```python
from build123d import *

# Parameters (mm, degrees)
F1_DEPTH = 50
F2_R     = 24.99999
F3_R     = 15.1938434026
F4_DEPTH = 73.4817621135
F5_R     = 5
F6_DEPTH = 38.6612540378


# Not quite as in the source:
# - a fillet or chamfer is up to 0.001 mm smaller than in the source, because OpenCascade refuses the exact size


with BuildPart() as f1:
    # F0 (on Top) → F1 (new body)
    with BuildSketch(Plane.XY):
        Polygon((0, 29.6784242139), (-80, 29.6784242139), (-80, 19.6784242139), (-2.6794919243, 19.6784242139), (46.9615242271, -8.9818298239), (51.9615242271, -0.3215757861), align=None)
    extrude(amount=F1_DEPTH)

    # F2 (radius 25 in the source; OpenCascade refuses exactly that, so slightly less here)
    f2_edges = [f1.edges().sort_by_distance(p)[0] for p in [
        (49.461524, -4.651703, 50),
        (49.461524, -4.651703, 0),
    ]]
    fillet(f2_edges, radius=F2_R)

    # F3 (on face) → F4 (cut, through all)
    with BuildSketch(Plane(origin=(12.8511346568, 22.2588181604, 0), x_dir=(-0.8660254038, 0.5, 0), z_dir=(0.5, 0.8660254038, 0))):
        with Locations((-20.160787893, 25)):
            Circle(F3_R)
    extrude(amount=-F4_DEPTH, mode=Mode.SUBTRACT)

    # F5 (on face) → F6 (cut, through all)
    with BuildSketch(Plane(origin=(0, 29.6784242139, 0), x_dir=(-1, 0, 0), z_dir=(0, 1, 0))):
        with Locations((12, 40)):
            Circle(F5_R)
        with Locations((70, 40)):
            Circle(F5_R)
        with Locations((12, 10)):
            Circle(F5_R)
        with Locations((70, 10)):
            Circle(F5_R)
    extrude(amount=-F6_DEPTH, mode=Mode.SUBTRACT)


solid = f1.part
```
Geometry: final body of the model. Coordinates: model frame, mm. A direction names the side the tool comes from. Coordinates: 2 decimals unless noted, no trailing zeros. Order: outer loops, then holes, each group sorted by start corner. A loop starts at its lowest first (then second) coordinate and runs counter-clockwise, first axis right, second up. Notation, with made-up numbers: (13.5, -8) -> (53.5, -8) arc R7 cw to (53.5, 5) -> close; hole circle Ø6 at (85, 20). An arc over 180 degrees is marked (long way). Write item = value, one per line.
(1) Pull-direction query (Z, two-part tool) for faces 1 (the flat face through (14.797, 21.135, 24.65)), 2 (the cylindrical face through (43.32, -1.03, 42.48)), 3 (the cylindrical face through (-74.619, 24.748, 8.085)); classes: pulls with the +Z half, pulls with the -Z half, needs draft (parallel to the pull), parting line crosses it, or undercut.
Solved:
face_1 = needs draft
face_2 = pulls with the +Z half
face_3 = undercut
(2) Line query: line 1 (Z direction, x = -70, y = 23); line 2 (Y direction, x = -28.5, z = 17.5); line 3 (Y direction, x = 13, z = 48.5). Output: solid intervals per line, ascending.
Solved:
line_1 = 0 to 5, 15 to 35, 45 to 50
line_2 = 19.68 to 29.68
line_3 = 10.63 to 22.17
(3) Cut plane A-A on x = -12. Return loops of the section in (y, z), plus the area to 3 significant figures.
Solved:
outline = (19.68, 0) -> (29.68, 0) -> (29.68, 5) -> (19.68, 5) -> close; (19.68, 15) -> (29.68, 15) -> (29.68, 35) -> (19.68, 35) -> close; (19.68, 45) -> (29.68, 45) -> (29.68, 50) -> (19.68, 50) -> close
area = 300 mm²
(4) Cut plane D-D on x = -63.5. Return loops of the section in (y, z), plus the area to 3 significant figures.
Solved:
outline = (19.68, 0) -> (29.68, 0) -> (29.68, 50) -> (19.68, 50) -> close
area = 500 mm²
(5) Access query for faces 4 (the flat face through (-26, 23, 0)), 5 (the flat face through (-42, 19.678, 25)). Directions: +Z, -Z, +X, -X, +Y, -Y. A direction counts if a zero-diameter tool reaches every point of the face in a straight line with its end or side. Return the directions, or none.
Solved:
face_4 = -Z, +X, -X, +Y, -Y
face_5 = +Z, -Z, -X, -Y
(6) Cut plane B-B on z = 18.5. Return loops of the section in (x, y).
Solved:
outline = (-80, 19.68) -> (-2.68, 19.68) -> (13.42, 10.38) -> (18.42, 19.05) -> (0, 29.68) -> (-80, 29.68) -> close; (37.2, -3.35) -> (46.22, -8.55) -> (51.22, 0.11) -> (42.2, 5.31) -> close
(7) Cut plane C-C on y = 24.5. Return loops of the section in (x, z).
Solved:
outline = (-80, 0) -> (8.97, 0) -> (8.97, 50) -> (-80, 50) -> close; hole circle Ø10 at (-70, 10); hole circle Ø10 at (-70, 40); hole circle Ø10 at (-12, 10); hole circle Ø10 at (-12, 40)
(8) Pin query (flat end, axial travel): pin 1 Ø13 at (x, z) = (-70, 10) entering from -Y; pin 2 Ø1 at (y, z) = (-1, 20) entering from +X; pin 3 Ø1 at (y, z) = (18.5, 16.5) entering from +X. Return the tip coordinate at first contact, or that it passes through.
Solved:
pin_1 = 19.68
pin_2 = 51.3
pin_3 = 19.69
